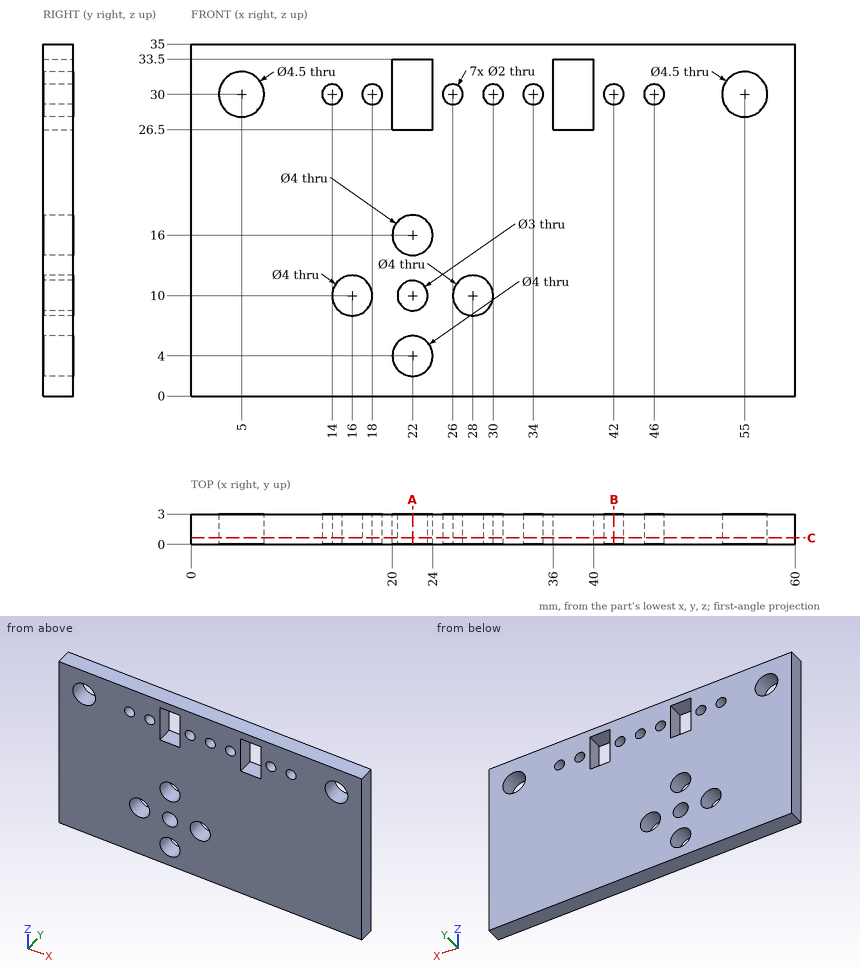
The drawing under review shows one solid part. Ordinate dimensions are in mm from its lowest x, y, z. Coordinates: 2 decimals unless noted, no trailing zeros. Order: outer loops, then holes, each group sorted by start corner. A loop starts at its lowest first (then second) coordinate and runs counter-clockwise, first axis right, second up. Notation, with made-up numbers: (61.5, -12) -> (65.5, -12) arc R14 ccw to (65.5, 0) -> close; hole circle Ø1 at (-36.75, 12). An arc over 180 degrees is marked (long way). One line per item, written item: value.
1) To check wall thickness, follow probe 1 along X at (y, z) = (1.2, 27.5); probe 2 along Z at (x, y) = (5, 1.55); probe 3 along Z at (x, y) = (16, 1.8). State the ranges of each line that lie inside material, in increasing order. Write a range as [from, to].
Output values:
probe 1: x = [0, 20], [24, 36], [40, 60]
probe 2: z = [0, 27.75], [32.25, 35]
probe 3: z = [0, 8], [12, 35]
2) Clearance check with a flat-ended pin moving along its axis: P1, Ø1.8, axis at x = 18, z = 30, coming from the +Y side. State where the tip first meets the part, or that it passes through.
Output values:
P1: passes through
3) We need section B-B, the plane x = 42. Give the boundary of the cut face in (y, z), then the cut area to 3 significant figures.
Output values:
outline: (0, 0) -> (3, 0) -> (3, 29) -> (0, 29) -> close; (0, 31) -> (3, 31) -> (3, 35) -> (0, 35) -> close
area: 99.0 mm2
4) We need section C-C, the plane y = 0.65. Count the separate pieces of the cut face and the enclosed holes in it, then the cut area to 3 significant figures.
Output values:
separate pieces: 1
enclosed holes: 16
area: 1,930 mm2
5) We need section A-A, the plane x = 22. Give the boundary of the cut face in (y, z), then the cut area to 3 significant figures.
Output values:
outline: (0, 0) -> (3, 0) -> (3, 2) -> (0, 2) -> close; (0, 6) -> (3, 6) -> (3, 8.5) -> (0, 8.5) -> close; (0, 11.5) -> (3, 11.5) -> (3, 14) -> (0, 14) -> close; (0, 18) -> (3, 18) -> (3, 26.5) -> (0, 26.5) -> close; (0, 33.5) -> (3, 33.5) -> (3, 35) -> (0, 35) -> close
area: 51.0 mm2
